Part model, mm, in its own coordinate system. Face numbers are marked on the shaded views. A direction names the side the tool comes from. Give positions to 0.01 mm unless a question says otherwise; leave off trailing zeros. Write each loop counter-clockwise with the first axis right and the second up, starting at its lowest first coordinate (ties: lowest second). Pieces come first, ordered by that corner, then holes. Notation, with made-up numbers: M 12.5,-8 L 40.5,-8 A29 cw 40.5,12 Z; hole C 1.5,27.5 d11. An arc over 180 degrees is marked long. Use CSV: the item, a comma, the result in double quotes. Start each with the question number.
1. Mould opens along Z. For the marked faces 1, 2 and 3 say: pulls with the +Z half, pulls with the -Z half, needs draft (parallel to the pull), parting line crosses it, or undercut.
2. Band-saw the part on C-C, the plane y = 17.5. List the corners of the cut face in (x, z).
3. Drop flat-ended pins along their axis: pin 1 Ø15.5 at (y, z) = (15, -30) entering from -X; pin 2 Ø2.5 at (x, z) = (17, -54.5) entering from +Y; pin 3 Ø1.5 at (y, z) = (29.5, -8.5) entering from +X; pin 4 Ø6 at (x, y) = (15, 13.5) entering from +Z. Give the stop position or say it passes through.
4. Band-saw the part on A-A, the plane x = 16. List the corners of the cut face in (y, z).
5. Drill centre lines: line 1 along Z through (x, y) = (16, 3.4); line 2 along Z through (x, y) = (3.75, 27.5); line 3 along X through (y, z) = (3.3, -4.5). Where is each one in solid material? Low to high. Write a range as from..to.
6. 3-axis set-ups, long thin cutter, end or side, ignore diameter. For the marked faces 4, 5 and 6: which of +Z, -Z, +X, -X, +Y, -Y reach the whole face in a straight line?
7. Band-saw the part on D-D, the plane z = -22. List the corners of the cut face in (x, y), then the cut area to 3 significant figures.
8. Band-saw the part on B-B, the plane z = -30. List the corners of the cut face in (x, y).
Autodesk Inventor part; units mm, degrees
ref_plane "YZ Plane" through (0, 0, 0) normal (1, 0, 0) x (0, 1, 0)
ref_plane "XZ Plane" through (0, 0, 0) normal (0, 1, 0) x (-1, 0, 0)
ref_plane "XY Plane" through (0, 0, 0) normal (0, 0, 1) x (1, 0, 0)
sketch "Boceto1" plane through (0, 0, 0) normal (1, 0, 0) x (0, 1, 0)
  line L0 (0, 0) -> (35, 0)
  line L1 (35, 0) -> (35, -60)
  line L2 (35, -60) -> (0, -60)
  line L3 (0, -60) -> (0, 0)
  circle A0 centre (15, -30) radius 6
  circle A1 centre (27.5, -17.5) radius 2
  circle A2 centre (27.5, -42.5) radius 2
  circle A3 centre (2.5, -42.5) radius 2
  circle A4 centre (2.5, -17.5) radius 2
  dimension "d0" = 60
  dimension "d1" = 35
  dimension "d2" = 20
  dimension "d3" = 30
  dimension "d4" = 12
  dimension "d5" = 12.5
  dimension "d6" = 12.5
  dimension "d7" = 12.5
  dimension "d8" = 12.5
  dimension "d9" = 12.5
  dimension "d10" = 12.5
  dimension "d11" = 12.5
  dimension "d12" = 12.5
  dimension "d13" = 4
  dimension "d14" = 4
  dimension "d15" = 4
  dimension "d16" = 4
extrude "Extrusión1" add sketch "Boceto1" along normal blind 10
sketch "Boceto3" plane through (10, 0, 0) normal (1, 0, 0) x (0, 0, -1)
  circle A0 centre (30, 15) radius 6
  circle A1 centre (30, 15) radius 22
  line L0 (0, 35) -> (0, 0)
  line L1 (0, 0) -> (9, 0)
  line L2 (9, 0) -> (9, 5)
  line L3 (9, 5) -> (0, 5)
  line L4 (0, 5) -> (0, 0)
  line L5 (0, 0) -> (60, 0)
  line L6 (60, 0) -> (51, 0)
  line L7 (51, 0) -> (51, 5)
  line L8 (51, 5) -> (60, 5)
  line L9 (60, 5) -> (60, 0)
  point P0 (0, 5)
  dimension "d19" = 44
  dimension "d20" = 9
  dimension "d21" = 5
  dimension "d22" = 9
  dimension "d23" = 5
extrude "Extrusión2" add sketch "Boceto3" along normal blind 10 contours L7 L8 L9 L5 | L1 L0 L3 L2
fillet "Empalme1" radius 2 4 edges at (10, 5, -4.5) (10, 5, -55.5) (10, 2.5, -9) (10, 2.5, -51)
sketch "Boceto4" plane through (20, 5, 0) normal (0, 1, 0) x (1, 0, 0)
  line L0 (-8, 9) -> (0, 9)
  line L1 (-8, 0) -> (0, 0)
  line L2 (-8, 60) -> (0, 60)
  line L3 (0, 9) -> (0, 0)
  line L4 (0, 60) -> (0, 51)
  point P0 (-20, 0)
  point P1 (-4, 4.5)
  point P2 (-4, 55.5)
  dimension "d27" = 4.5
  dimension "d28" = 9
  dimension "d29" = 4.5
  dimension "d30" = 4
  dimension "d31" = 4
hole "Agujero1" at (16, 5, -4.5) at (16, 5, -55.5) direction (0, -1, 0) diameter 5 end through all
fillet "Empalme2" radius 8 2 edges at (5, 35, 0) (5, 35, -60)
sketch "Boceto5" plane through (0, 0, 0) normal (-1, 0, 0) x (0, 0, 1)
  circle A0 centre (-30, 15) radius 6
  circle A1 centre (-30, 15) radius 13
  point P0 (0, 0)
  dimension "d40" = 26
extrude "Extrusión3" cut sketch "Boceto5" against normal blind 2.6
fillet "Empalme3" radius 2 4 edges at (20, 2.5, 0) (20, 2.5, -9) (20, 2.5, -51) (20, 2.5, -60)
equation "\"d3\" = 0.5 * d0"
equation "\"d6\" = d5"
equation "\"d7\" = d5"
equation "\"d8\" = d5"
equation "\"d9\" = d5"
equation "\"d10\" = d5"
equation "\"d11\" = d5"
equation "\"d12\" = d5"
equation "\"d14\" = d13"
equation "\"d15\" = d13"
equation "\"d16\" = d13"
equation "\"d22\" = d20"
properties part number "Soporte_motor_aluminio"
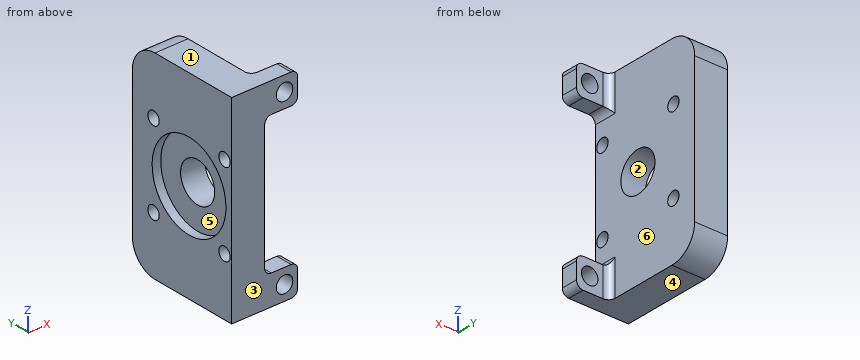
Output:
1,face 1,"pulls with the +Z half"
1,face 2,"undercut"
1,face 3,"needs draft"
2,outline,"M 0,-60 L 10,-60 L 10,-35.45 L 2.6,-35.45 L 2.6,-42.76 L 0,-42.76 Z; M 0,-17.24 L 2.6,-17.24 L 2.6,-24.55 L 10,-24.55 L 10,0 L 0,0 Z"
3,pin 1,"stops at x = 2.6"
3,pin 2,"stops at y = 5"
3,pin 3,"stops at x = 10"
3,pin 4,"passes through"
4,outline,"M 0,-60 L 5,-60 L 5,-58 L 0,-58 Z; M 0,-53 L 5,-53 L 5,-51 L 0,-51 Z; M 0,-9 L 5,-9 L 5,-7 L 0,-7 Z; M 0,-2 L 5,-2 L 5,0 L 0,0 Z"
5,line 1,"z = -60..-58, -53..-51, -9..-7, -2..0"
5,line 2,"z = -59.98..-44.5, -40.5..-19.5, -15.5..-0.02"
5,line 3,"x = 0..13.5, 18.5..20"
6,face 4,"-Z, +X, -X, +Y, -Y"
6,face 5,"-X"
6,face 6,"+X, +Y"
7,outline,"M 0,0 L 10,0 L 10,35 L 0,35 L 0,25.25 L 2.6,25.25 L 2.6,4.75 L 0,4.75 Z"
7,area,"297 mm²"
8,outline,"M 0,0 L 10,0 L 10,9 L 2.6,9 L 2.6,2 L 0,2 Z; M 0,28 L 2.6,28 L 2.6,21 L 10,21 L 10,35 L 0,35 Z"
